Source: CAD feature listing. Evaluate the final solid. Frame: model axes, mm. Round coordinates to 2 decimals unless told otherwise and drop trailing zeros. Loops run counter-clockwise (first coordinate to the right, second up) from the corner with the lowest first, then second, coordinate; pieces in that order, holes last. Notation, with made-up numbers: M 81.25,27.5 L 110.25,27.5 A18 ccw 110.25,59.5 Z; hole C 20.25,88 d2. An arc over 180 degrees is marked long. Answer as CSV lines item,"result". Start each with the question number.
```python
from build123d import *

# Parameters (mm, degrees)
SALIENTE_EXTRUIR1_DEPTH = 1.875
CROQUIS2_R              = 0.225
CORTAR_EXTRUIR1_DEPTH   = 0.3


with BuildPart() as part:
    # Croquis1 → Saliente-Extruir1 (new, symmetric)
    with BuildSketch(Plane.XY):
        with BuildLine():
            Line((4.537261216, -15.5500625), (-7.929262831, -17.609800574))
            Line((-7.929262831, -17.609800574), (-7.9048111, -17.757794198))
            Line((-7.9048111, -17.757794198), (4.561712947, -15.698056124))
            ThreePointArc((4.561712947, -15.698056124), (4.651774684, -15.643632038), (4.699918625, -15.5500625))
            Line((4.699918625, -15.5500625), (4.537261216, -15.5500625))
        make_face()
    extrude(amount=SALIENTE_EXTRUIR1_DEPTH, both=True)

    # Croquis2 → Cortar-Extruir1 (cut)
    with BuildSketch(Plane(origin=(2.645953415, -16.01458083, 0), x_dir=(0.9866241615125322, 0.16301154535704834, 0), z_dir=(0.16301154535704834, -0.9866241615125322, 0))):
        with Locations((-4.376035637, 1.875)):
            Circle(CROQUIS2_R)
        with Locations((-4.376035637, -1.875)):
            Circle(CROQUIS2_R)
        with BuildLine():
            Line((9.881731824, -0.5), (-5.518268176, -0.5))
            ThreePointArc((-5.518268176, -0.5), (-5.857679431, -0.359411255), (-5.998268176, -0.02))
            Line((-5.998268176, -0.02), (-5.998268176, 0.02))
            ThreePointArc((-5.998268176, 0.02), (-5.857679431, 0.359411255), (-5.518268176, 0.5))
            Line((-5.518268176, 0.5), (9.881731824, 0.5))
            Line((9.881731824, 0.5), (9.881731824, -0.5))
        make_face()
    extrude(amount=-CORTAR_EXTRUIR1_DEPTH, mode=Mode.SUBTRACT)


solid = part.part
```
1) Section B-B, the plane y = -16.15. Return loops of the section in (x, z) (3 decimals).
2) Contact query for a flat-ended pin moving along its axis: pin 1 Ø1 at (x, z) = (-4, -0.5) entering from +Y. Output: stop coordinate, or through.
3) Section A-A, the plane x = 1.75. Return loops of the section in (y, z) (3 decimals), and give its area (3 significant figures).
4) Section D-D, the plane y = -17.3. Return loops of the section in (x, z) (3 decimals), and give its area (3 significant figures).
5) Ray query, line 1 along Y through (x, z) = (2.5, -1.7); line 2 along Y through (x, z) = (0.75, -1.2). Return the intervals inside material, ascending.
6) Section C-C, the plane z = -1.2. Return loops of the section in (x, y).
Findings below:
1,outline,"M 0.906,-1.875 L 1.826,-1.875 L 1.826,-0.5 L 0.906,-0.5 Z; M 0.906,0.5 L 1.826,0.5 L 1.826,1.875 L 0.906,1.875 Z"
2,pin 1,"y = -16.88"
3,outline,"M -16.163,-1.875 L -16.011,-1.875 L -16.011,-0.5 L -16.163,-0.5 Z; M -16.163,0.5 L -16.011,0.5 L -16.011,1.875 L -16.163,1.875 Z"
3,area,"0.418 mm²"
4,outline,"M -6.054,-1.875 L -5.134,-1.875 L -5.134,1.875 L -6.054,1.875 Z"
4,area,"3.45 mm²"
5,line 1,"-16.04 to -15.89"
5,line 2,"-16.33 to -16.18"
6,outline,"M -7.93,-17.61 L -7.9,-17.76 L 4.56,-15.7 A0.19 ccw 4.7,-15.55 L 4.54,-15.55 Z"
